Answer from the drawing. Dimensions are ordinates in mm from the lowest x, y and z of the part. A direction names the side the tool comes from. Give positions to 0.01 mm unless a question says otherwise; leave off trailing zeros. Loops run counter-clockwise (first coordinate to the right, second up) from the corner with the lowest first, then second, coordinate; pieces in that order, holes last. Notation, with made-up numbers: (-36.5, -38.5) - (-7.5, -38.5) arc R17 ccw to (-7.5, -24.5) - close; hole circle Ø6 at (55.5, 20). An arc over 180 degrees is marked (long way). Answer as CSV lines item,"result". Start each with the question number.
1) For a pull along X with two mould halves and no side action, classify the marked faces 3, 4 and 5 as pulls with the +X half, pulls with the -X half, needs draft (parallel to the pull), parting line crosses it, or undercut.
2) Find the intervals of material crossed by line 1 along X through (y, z) = (57, 40); line 2 along Y through (x, z) = (129.5, 32); line 3 along Z through (x, y) = (116, 82.5), in increasing order.
3) For the marked faces 1 and 2, determine the directions among +Z, -Z, +X, -X, +Y, -Y from which every point of the face is accessible in a straight line to the end or side of a thin tool.
4) A cutting plane is placed at A-A (z = 39.5). Determine the outline of the cut face in (x, y).
5) Flat-ended cylindrical pins translate along their axes: pin 1 (19 mm diameter, centred on y = 50.5, z = 39, fed in from -X); pin 2 (5 mm diameter, centred on x = 45.5, y = 54, fed in from +Z). Find the tip coordinate at first contact, or state that the pin passes through.
6) A cutting plane is placed at B-B (x = 67). Determine the outline of the cut face in (y, z).
7) A cutting plane is placed at C-C (y = 98). Determine the outline of the cut face in (x, z).
8) A cutting plane is placed at D-D (z = 27). Determine the outline of the cut face in (x, y).
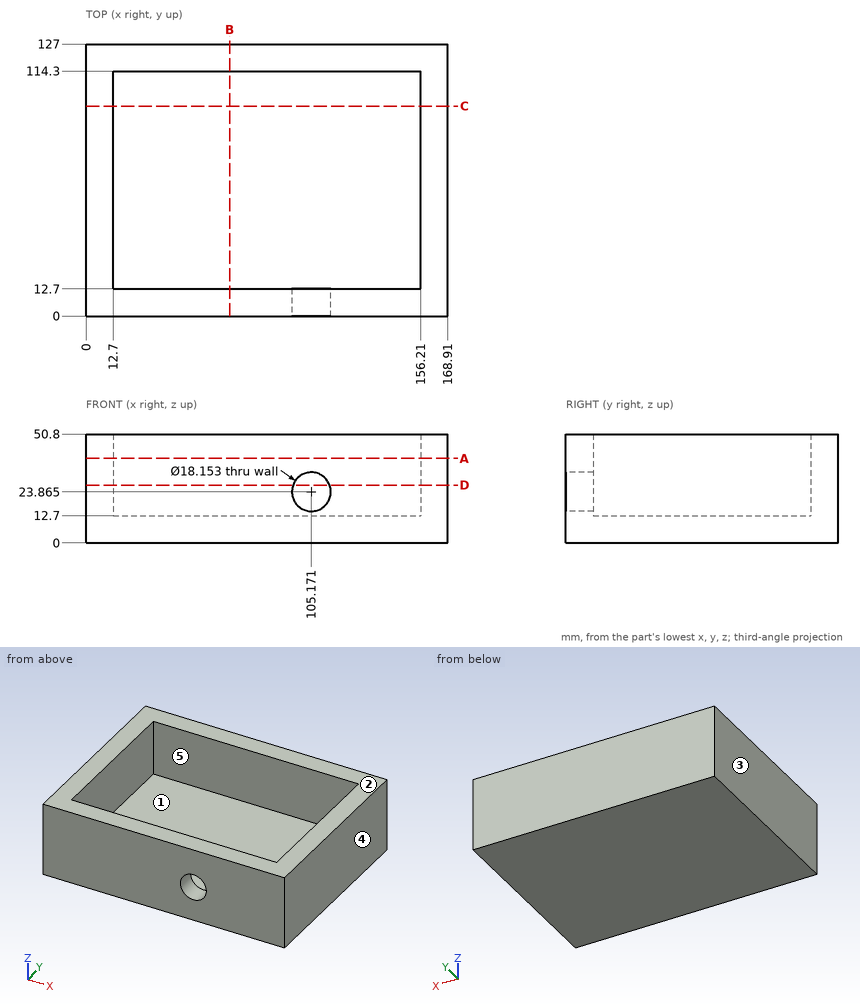
Ans:
1,face 3,"pulls with the -X half"
1,face 4,"pulls with the +X half"
1,face 5,"undercut"
2,line 1,"0 to 12.7, 156.21 to 168.91"
2,line 2,"0 to 12.7, 114.3 to 127"
2,line 3,"0 to 12.7"
3,face 1,"+Z"
3,face 2,"+Z, +X, -X, +Y, -Y"
4,outline,"(0, 0) - (168.91, 0) - (168.91, 127) - (0, 127) - close; hole (12.7, 12.7) - (156.21, 12.7) - (156.21, 114.3) - (12.7, 114.3) - close"
5,pin 1,"x = 0"
5,pin 2,"z = 12.7"
6,outline,"(0, 0) - (127, 0) - (127, 50.8) - (114.3, 50.8) - (114.3, 12.7) - (12.7, 12.7) - (12.7, 50.8) - (0, 50.8) - close"
7,outline,"(0, 0) - (168.91, 0) - (168.91, 50.8) - (156.21, 50.8) - (156.21, 12.7) - (12.7, 12.7) - (12.7, 50.8) - (0, 50.8) - close"
8,outline,"(0, 0) - (96.65, 0) - (96.65, 12.7) - (12.7, 12.7) - (12.7, 114.3) - (156.21, 114.3) - (156.21, 12.7) - (113.69, 12.7) - (113.69, 0) - (168.91, 0) - (168.91, 127) - (0, 127) - close"
